Geometry check sheet. Reference: the model listing, model coordinates, mm. A direction names the side the tool comes from. Give positions to 0.01 mm unless a question says otherwise; leave off trailing zeros. Loops run counter-clockwise (first coordinate to the right, second up) from the corner with the lowest first, then second, coordinate; pieces in that order, holes last. Notation, with made-up numbers: (20.5, 72.5) -> (43.5, 72.5) arc R20 ccw to (43.5, 83.5) -> close; hole circle Ø2 at (45.5, 4). An arc over 180 degrees is marked (long way). Write item = value, one per line.
```python
from build123d import *

# Parameters (mm, degrees)
SKETCH_1_R          = 1.95
EXTRUDE_1_DEPTH     = 12
SKETCH_4_W          = 2
SKETCH_4_H          = 9
EXTRUDE_2_DEPTH     = 1.95
EXTRUDE_4_DEPTH     = 8.8
SKETCH_9_R          = 1
CUT_EXTRUDE_2_DEPTH = 17
SKETCH_13_R         = 1.375
CUT_EXTRUDE_6_DEPTH = 1
CUT_EXTRUDE_7_DEPTH = 13.389713
SCALE_1_SCALE       = 2


with BuildPart() as part:
    # 스케치1 → 보스-돌출1 (new body)
    with BuildSketch(Plane.XY):
        Circle(SKETCH_1_R)
    extrude(amount=EXTRUDE_1_DEPTH)

    # 스케치4 → 보스-돌출2 (add)
    with BuildSketch(Plane(origin=(0, 0, 0), x_dir=(0, 0, -1), z_dir=(1, 0, 0))):
        with Locations((-1, -2.55)):
            Rectangle(SKETCH_4_W, SKETCH_4_H)
    extrude(amount=EXTRUDE_2_DEPTH)

    # 스케치8 → 보스-돌출4 (add)
    with BuildSketch(Plane.XY.offset(2)):
        with BuildLine():
            ThreePointArc((1.95, -1.643168), (1.075273, -2.312204), (0, -2.55))
            Line((0, -2.55), (0, -7.05))
            Line((0, -7.05), (1.95, -7.05))
            Line((1.95, -7.05), (1.95, -1.643168))
        make_face()
    extrude(amount=EXTRUDE_4_DEPTH)

    # 스케치9 → 컷-돌출2 (cut)
    with BuildSketch(Plane.ZY):
        with Locations((5.5, -7.55)):
            Circle(SKETCH_9_R)
    extrude(amount=-CUT_EXTRUDE_2_DEPTH, mode=Mode.SUBTRACT)

    # 스케치13 → 컷-돌출6 (cut)
    with BuildSketch(Plane.ZY):
        with Locations((5.505014, -7.55)):
            Circle(SKETCH_13_R)
    extrude(amount=-CUT_EXTRUDE_6_DEPTH, mode=Mode.SUBTRACT)

    # 스케치12 → 컷-돌출7 (cut, through all)
    with BuildSketch(Plane.XY.offset(2)):
        with BuildLine():
            Line((1.95, 0), (1.95, 1.95))
            Line((1.95, 1.95), (0, 1.95))
            ThreePointArc((0, 1.95), (1.378858, 1.378858), (1.95, 0))
        make_face()
    extrude(amount=-CUT_EXTRUDE_7_DEPTH, mode=Mode.SUBTRACT)


with BuildPart() as part_1:
    # 축척1: scaled about (0, 0, 0)
    add(part.part.scale(SCALE_1_SCALE))


solid = part_1.part
```
Item 1: Draft check along X on faces 1 (the flat face through (2, -14.1, 5)), 2 (the flat face through (3.9, -9, 11)), 3 (the flat face through (2, -4, 4)). Enter one of: +X half, -X half, draft (parallel to the pull), parting line (faces both ways), or undercut.
Answer:
face_1 = draft
face_2 = +X half
face_3 = undercut
Item 2: Gauge pin test, flat ends, axial feed: pin 1 (4 mm diameter, centred on x = 2.5, y = -11.5, fed in from -Z); pin 2 (0.5 mm diameter, centred on y = -13.5, z = 12, fed in from -X); pin 3 (3 mm diameter, centred on y = -8.5, z = 6.5, fed in from -X); pin 4 (3 mm diameter, centred on x = 1.5, y = -8, fed in from +Z). Record the tip position at first contact, or that the pin passes through.
Answer:
pin_1 = 0
pin_2 = 2
pin_3 = 0
pin_4 = 21.6
Item 3: Section check D-D, the plane z = 22.25. Record the cut outline in (x, y).
Answer:
outline = circle Ø7.8 at (0, 0)
Item 4: Section check C-C, the plane x = 1. Record the cut outline in (y, z), plus the area to 3 significant figures.
Answer:
outline = (-14.1, 0) -> (3.77, 0) -> (3.77, 24) -> (-3.77, 24) -> (-3.77, 4) -> (-5, 4) -> (-5, 21.6) -> (-14.1, 21.6) -> (-14.1, 13.57) arc R2.75 cw to (-14.1, 8.45) -> close
area = 376 mm^2
Item 5: Section check B-B, the plane y = -1.5. Record the cut outline in (x, z).
Answer:
outline = (-3.6, 0) -> (3.9, 0) -> (3.9, 4) -> (3.6, 4) -> (3.6, 24) -> (-3.6, 24) -> close
Item 6: Tool access check on faces 4 (the cylindrical face through (0.99, -12.35, 11.06)), 5 (the flat face through (0, -9, 11)), 6 (the cylindrical face through (2.2, -4.6, 12.7)), 7 (the flat face through (2, -14.1, 17)), 8 (the flat face through (1, -3, 0)). Record the directions out of +Z, -Z, +X, -X, +Y, -Y that give a thin tool (end or side, any length) a straight path to the whole face; none if there is none.
Answer:
face_4 = -X, -Y
face_5 = +Z, -Z, -X, -Y
face_6 = +Z
face_7 = +Z, -Z, +X, -X, -Y
face_8 = -Z, +X, -X, +Y, -Y
Item 7: Section check A-A, the plane z = 8. Record the cut outline in (x, y).
Answer:
outline = circle Ø7.8 at (0, 0); (0, -14.1) -> (3.9, -14.1) -> (3.9, -3.29) arc R5.1 cw to (0, -5.1) -> close
Item 8: Thickness scan on L1, parallel to X at y = -11.75, z = 9; L2, parallel to Y at x = 1.75, z = 15; L3, parallel to Z at x = 2.5, y = -7. Record the ranges inside material, lowest first. Write a range as [from, to].
Answer:
L1 = [0, 3.9]
L2 = [-14.1, -4.79], [-3.49, 3.49]
L3 = [0, 21.6]
